Geometry: see drawing. Coordinates: mm, zero at the bounding-box minimum. A direction names the side the tool comes from. Give positions to 0.01 mm unless a question says otherwise; leave off trailing zeros. Order: outer loops, then holes, each group sorted by start corner. A loop starts at its lowest first (then second) coordinate and runs counter-clockwise, first axis right, second up. Notation, with made-up numbers: (17.25, 89.25) - (62.25, 89.25) arc R28 cw to (62.25, 125.25) - close; hole circle Ø7 at (9, -35). An arc over 180 degrees is marked (long way). One line per item, written item: value.
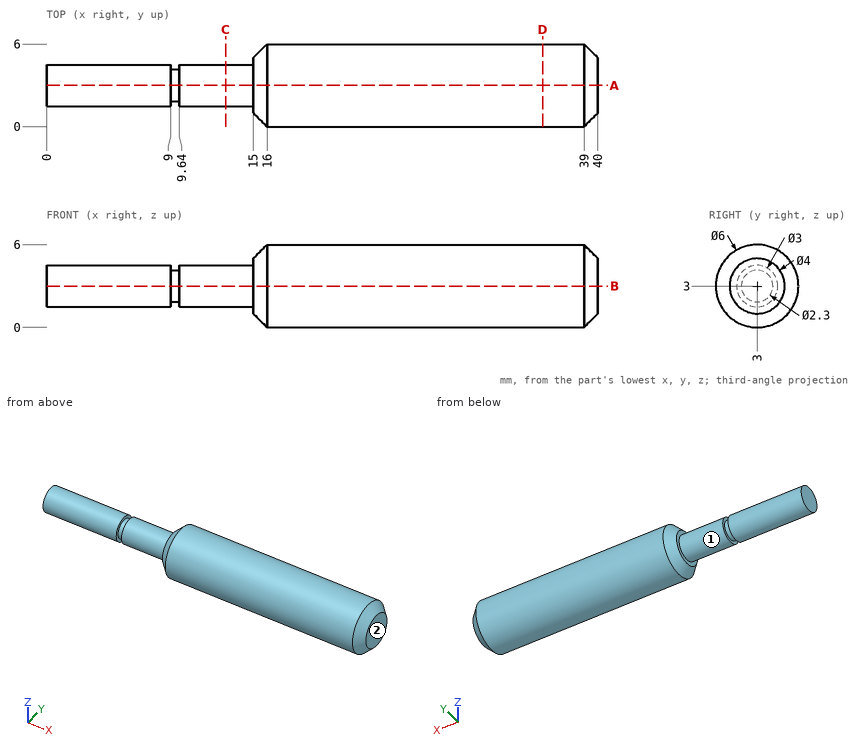
1) Material intervals for line 1 along X through (y, z) = (2.2, 3.9); line 2 along Y through (x, z) = (29.5, 2.85); line 3 along X through (y, z) = (1.2, 3.4), sorted ascending.
Answers below:
line 1: 0 to 9, 9.64 to 40
line 2: 0 to 6
line 3: 15 to 40
2) First-contact query: pin 1 (1 mm diameter, centred on x = 34.5, z = 5, fed in from +Y); pin 2 (1.5 mm diameter, centred on x = 5, z = 0.5, fed in from +Y); pin 3 (2 mm diameter, centred on x = 30, z = 1.5, fed in from -Y). Flat tips, straight axial feed; report the tip coordinate or a pass-through.
Answers below:
pin 1: y = 5.6
pin 2: through
pin 3: y = 0.04
3) Set-up query: the marked faces 1 and 2. Return all of +Z, -Z, +X, -X, +Y, -Y with unobstructed straight access to the full face (end or side cutting, diameter ignored); none if empty.
Answers below:
face 1: -X
face 2: +Z, -Z, +X, +Y, -Y
4) Section D-D, the plane x = 36. Return loops of the section in (y, z).
Answers below:
outline: circle Ø6 at (3, 3)
5) Section C-C, the plane x = 13. Return loops of the section in (y, z).
Answers below:
outline: circle Ø3 at (3, 3)
6) Section A-A, the plane y = 3. Return loops of the section in (x, z).
Answers below:
outline: (0, 1.5) - (9, 1.5) - (9, 1.85) - (9.64, 1.85) - (9.64, 1.5) - (15, 1.5) - (15, 1) - (16, 0) - (39, 0) - (40, 1) - (40, 5) - (39, 6) - (16, 6) - (15, 5) - (15, 4.5) - (9.64, 4.5) - (9.64, 4.15) - (9, 4.15) - (9, 4.5) - (0, 4.5) - close
